Model file for the job. Use its own axes, mm. Face numbers are marked on the shaded views. A direction names the side the tool comes from. Round coordinates to 2 decimals unless told otherwise and drop trailing zeros. Write each loop counter-clockwise with the first axis right and the second up, starting at its lowest first coordinate (ties: lowest second). Pieces come first, ordered by that corner, then holes. Notation, with made-up numbers: (55.5, 33) - (96.5, 33) arc R34 ccw to (96.5, 69) - close; hole circle Ø3 at (60.5, 46.5). An arc over 180 degrees is marked (long way). Answer as a JSON object with one key per item and string values. Group by question number.
from build123d import *

# Parameters (mm, degrees)
SKETCH1_W           = 22.75
SKETCH1_H           = 12.25
BOSS_EXTRUDE1_DEPTH = 16.75
BOSS_EXTRUDE2_DEPTH = 2.5
CUT_EXTRUDE1_DEPTH  = 1
SKETCH5_W           = 22.75
SKETCH5_H           = 12.25
BOSS_EXTRUDE3_DEPTH = 4
BOSS_EXTRUDE4_DEPTH = 4.5
SKETCH7_R           = 2.375
SKETCH7_R_2         = 0.875
BOSS_EXTRUDE5_DEPTH = 2.75
BOSS_EXTRUDE6_DEPTH = 4


with BuildPart() as part:
    # Sketch1 → Boss-Extrude1 (new body)
    with BuildSketch(Plane(origin=(0, 0, 0), x_dir=(1, 0, 0), z_dir=(0, 1, 0))):
        Rectangle(SKETCH1_W, SKETCH1_H)
    extrude(amount=BOSS_EXTRUDE1_DEPTH)

    # Sketch3 → Boss-Extrude2 (add)
    with BuildSketch(Plane(origin=(0, 16.75, 0), x_dir=(1, 0, 0), z_dir=(0, 1, 0))):
        with BuildLine():
            Line((-16.15, -6.125), (16.15, -6.125))
            Line((16.15, -6.125), (16.15, -0.6))
            Line((16.15, -0.6), (14.84658561, -0.6))
            ThreePointArc((14.84658561, -0.6), (12.5, 0), (14.84658561, 0.6))
            Line((14.84658561, 0.6), (16.15, 0.6))
            Line((16.15, 0.6), (16.15, 6.125))
            Line((16.15, 6.125), (-16.15, 6.125))
            Line((-16.15, 6.125), (-16.15, 0.6))
            Line((-16.15, 0.6), (-14.84658561, 0.6))
            ThreePointArc((-14.84658561, 0.6), (-12.5, 0), (-14.84658561, -0.6))
            Line((-14.84658561, -0.6), (-16.15, -0.6))
            Line((-16.15, -0.6), (-16.15, -6.125))
        make_face()
    extrude(amount=BOSS_EXTRUDE2_DEPTH)

    # Sketch4 → Cut-Extrude1 (cut)
    with BuildSketch(Plane.XZ.offset(-16.75)):
        with BuildLine():
            Line((-11.375, -5.125), (-15.15, -5.125))
            Line((-15.15, -5.125), (-15.15, -1.761391495))
            ThreePointArc((-15.15, -1.761391495), (-11.5, 0), (-15.15, 1.761391495))
            Line((-15.15, 1.761391495), (-15.15, 5.125))
            Line((-15.15, 5.125), (-11.375, 5.125))
            Line((-11.375, 5.125), (-11.375, -5.125))
        make_face()
        with BuildLine():
            Line((11.375, 5.125), (11.375, -5.125))
            Line((11.375, -5.125), (15.15, -5.125))
            Line((15.15, -5.125), (15.15, -1.761391495))
            ThreePointArc((15.15, -1.761391495), (11.5, 0), (15.15, 1.761391495))
            Line((15.15, 1.761391495), (15.15, 5.125))
            Line((15.15, 5.125), (11.375, 5.125))
        make_face()
    extrude(amount=-CUT_EXTRUDE1_DEPTH, mode=Mode.SUBTRACT)

    # Sketch5 → Boss-Extrude3 (add)
    with BuildSketch(Plane(origin=(0, 19.25, 0), x_dir=(1, 0, 0), z_dir=(0, 1, 0))):
        Rectangle(SKETCH5_W, SKETCH5_H)
    extrude(amount=BOSS_EXTRUDE3_DEPTH)

    # Sketch6 → Boss-Extrude4 (add)
    with BuildSketch(Plane(origin=(0, 23.25, 0), x_dir=(1, 0, 0), z_dir=(0, 1, 0))):
        with BuildLine():
            Line((-0.575, 2.8), (-0.197533846, 2.8))
            ThreePointArc((-0.197533846, 2.8), (11.375, 0), (-0.197533846, -2.8))
            Line((-0.197533846, -2.8), (-0.575, -2.8))
            ThreePointArc((-0.575, -2.8), (-3.375, 0), (-0.575, 2.8))
        make_face()
    extrude(amount=BOSS_EXTRUDE4_DEPTH)

    # Sketch7 → Boss-Extrude5 (add)
    with BuildSketch(Plane(origin=(0, 27.75, 0), x_dir=(1, 0, 0), z_dir=(0, 1, 0))):
        with Locations((5.25, 0)):
            Circle(SKETCH7_R)
        with Locations((5.25, 0)):
            Circle(SKETCH7_R_2, mode=Mode.SUBTRACT)
    extrude(amount=BOSS_EXTRUDE5_DEPTH)

    # Sketch8 → Boss-Extrude6 (add)
    with BuildSketch(Plane(origin=(11.375, 0, 0), x_dir=(0, 0, -1), z_dir=(1, 0, 0))):
        with BuildLine():
            Line((-1.25, 2), (1.25, 2))
            ThreePointArc((1.25, 2), (2, 1.25), (1.25, 0.5))
            Line((1.25, 0.5), (-1.25, 0.5))
            ThreePointArc((-1.25, 0.5), (-2, 1.25), (-1.25, 2))
        make_face()
    extrude(amount=BOSS_EXTRUDE6_DEPTH)


solid = part.part
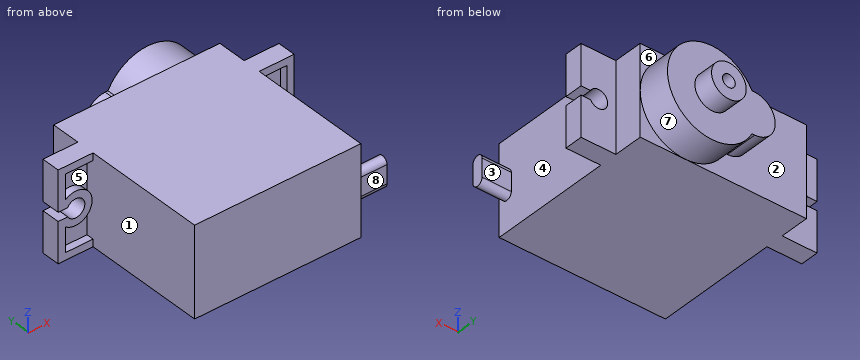
(1) Drill centre lines: line 1 (Z direction, x = -13.75, y = 17.7) (3 decimals); line 2 (X direction, y = 17.5, z = 3) (3 decimals); line 3 (X direction, y = 29.95, z = 0) (3 decimals). Where is each one in solid material? Low to high. Write a range as from..to.
(2) Flat gauge pins, fed straight in: pin 1 (3 mm diameter, centred on y = 6, z = 3, fed in from +X) (3 decimals); pin 2 (3 mm diameter, centred on x = 9, z = 3, fed in from +Y); pin 3 (3 mm diameter, centred on x = -14, z = 1, fed in from -Y); pin 4 (1.4 mm diameter, centred on x = -13.5, z = 0, fed in from -Y). Where does each tip first touch, or does it go through?
(3) Slice it at C-C (x = 10.5). Write the cut outline in (y, z) (3 decimals), then the cut area to 3 significant figures.
(4) Pull direction Y, two halves, no side cores. Call the marked faces 1, 2, 3 and 4: pulls with the +Y half, pulls with the -Y half, needs draft (parallel to the pull), parting line crosses it, or undercut.
(5) Slice it at A-A (x = -13.75). Write the cut outline in (y, z) (3 decimals).
(6) Slice it at B-B (y = 1.25). Write the cut outline in (x, z) (3 decimals).
(7) 3-axis set-ups, long thin cutter, end or side, ignore diameter. For the marked faces 5, 6, 7 and 8: which of +Z, -Z, +X, -X, +Y, -Y reach the whole face in a straight line?
Answer:
{
 "1": {"line 1": "-6.125..-5.125, -2.25..-1.25, 1.25..2.25, 5.125..6.125", "line 2": "-16.15..-15.15, -11.375..11.375, 15.15..16.15", "line 3": "2.875..4.375, 6.125..7.625"},
 "2": {"pin 1": "x = 11.375", "pin 2": "y = 27.75", "pin 3": "y = 16.75", "pin 4": "through"},
 "3": {"outline": "(0, -6.125) - (23.25, -6.125) - (23.25, -3.155) - (27.75, -3.155) - (27.75, 3.155) - (23.25, 3.155) - (23.25, 6.125) - (0, 6.125) - close", "area": "313 mm²"},
 "4": {"face 1": "needs draft", "face 2": "pulls with the +Y half", "face 3": "undercut", "face 4": "undercut"},
 "5": {"outline": "(16.75, -6.125) - (19.25, -6.125) - (19.25, -1.25) - (16.75, -1.25) - (16.75, -2.25) - (17.75, -2.25) - (17.75, -5.125) - (16.75, -5.125) - close; (16.75, 1.25) - (19.25, 1.25) - (19.25, 6.125) - (16.75, 6.125) - (16.75, 5.125) - (17.75, 5.125) - (17.75, 2.25) - (16.75, 2.25) - close"},
 "6": {"outline": "(-11.375, -6.125) - (11.375, -6.125) - (11.375, -2) - (15.375, -2) - (15.375, 2) - (11.375, 2) - (11.375, 6.125) - (-11.375, 6.125) - close"},
 "7": {"face 5": "-Y", "face 6": "+Z, +X, +Y", "face 7": "+Y", "face 8": "+Z, -Z, +X, -Y"}
}
